Autodesk Fusion 360 part; units mm, degrees
sketch "Sketch1" plane through (0, 0, 0) normal (0, 0, 1) x (1, 0, 0)
  line L0 (12.2, 9.5) -> (-12.2, 9.5)
  line L1 (-12.2, 9.5) -> (-12.2, -9.5)
  line L2 (-12.2, -9.5) -> (12.2, -9.5)
  line L3 (12.2, -9.5) -> (12.2, 9.5)
  line L4 (12.2, 9.5) -> (-12.2, -9.5) construction
  line L5 (-12.2, 9.5) -> (12.2, -9.5) construction
  line L6 (9.2, 6.5) -> (-9.2, 6.5) construction
  line L7 (-9.2, 6.5) -> (-9.2, -6.5) construction
  line L8 (-9.2, -6.5) -> (9.2, -6.5) construction
  line L9 (9.2, -6.5) -> (9.2, 6.5) construction
  line L10 (9.2, 6.5) -> (-9.2, -6.5) construction
  line L11 (-9.2, 6.5) -> (9.2, -6.5) construction
  circle A0 centre (9.2, 6.5) radius 1.5
  circle A1 centre (-9.2, -6.5) radius 1.5
  line L12 (0, 0) -> (9.2, 0) construction
  circle A2 centre (-9.2, 6.5) radius 1.5
  circle A3 centre (9.2, -6.5) radius 1.5
  line L13 (6.2, 7.5) -> (-6.2, 7.5)
  line L14 (-6.2, 7.5) -> (-6.2, -7.5)
  line L15 (-6.2, -7.5) -> (6.2, -7.5)
  line L16 (6.2, -7.5) -> (6.2, 7.5)
  line L17 (6.2, 7.5) -> (-6.2, -7.5) construction
  line L18 (-6.2, 7.5) -> (6.2, -7.5) construction
  line L19 (0, 0) -> (5.0501, 0) construction
  line L20 (19.3001, 18.69) -> (-9.2, 18.69) construction
  line L21 (-9.2, 18.69) -> (-9.2, -18.69) construction
  line L22 (-9.2, -18.69) -> (19.3001, -18.69) construction
  line L23 (19.3001, -18.69) -> (19.3001, 18.69) construction
  line L24 (19.3001, 18.69) -> (-9.2, -18.69) construction
  line L25 (-9.2, 18.69) -> (19.3001, -18.69) construction
  circle A4 centre (-9.2, 18.69) radius 1.5
  circle A5 centre (-9.2, -18.69) radius 1.5
  line L26 (-12.2, 21.69) -> (-4.2, 21.69)
  line L27 (-4.2, 21.69) -> (-4.2, -21.69)
  line L28 (-4.2, -21.69) -> (-12.2, -21.69)
  line L29 (-12.2, -21.69) -> (-12.2, 21.69)
  point P0 (5.0501, 0)
  dimension "d1" = 18.4
  dimension "d2" = 13
  dimension "d3" = 3
  dimension "d6" = 3
  dimension "d7" = 3
  dimension "d10" = 3
  dimension "d11" = 2
  dimension "d14" = 37.38
  dimension "d15" = 3
  dimension "d16" = 3
  dimension "d17" = 5
  dimension "d18" = 3
  dimension "d19" = 3
extrude "Extrude1" add sketch "Sketch1" along normal blind 12 contours L0 L2 L3 L13 L15 L16 L27 | L0 L1 L2 L13 L14 L15 L27 L29
fillet "Fillet1" radius 2 4 edges at (12.2, -9.5, 6) (12.2, 9.5, 6) (-12.2, 9.5, 6) (-12.2, -9.5, 6)
thread "Thread1"
sketch "Sketch2" plane through (0, 0, 12) normal (0, 0, 1) x (1, 0, 0)
  line L0 (-12.2, 7.5) -> (-12.2, -7.5)
  line L1 (-10.2, -9.5) -> (10.2, -9.5)
  arc A0 (10.2, -9.5) -> (12.2, -7.5) centre (10.2, -7.5) ccw
  line L2 (12.2, -7.5) -> (12.2, 7.5)
  arc A1 (12.2, 7.5) -> (10.2, 9.5) centre (10.2, 7.5) ccw
  line L3 (10.2, 9.5) -> (-10.2, 9.5)
  line L4 (6.2, 7.5) -> (6.2, -7.5)
  line L5 (6.2, -7.5) -> (-6.2, -7.5)
  line L6 (-6.2, -7.5) -> (-6.2, 7.5)
  line L7 (-6.2, 7.5) -> (6.2, 7.5)
  circle A2 centre (9.2, 6.5) radius 1.2645
  circle A3 centre (-9.2, -6.5) radius 1.2645
  circle A4 centre (9.2, -6.5) radius 1.2645
  circle A5 centre (-9.2, 6.5) radius 1.2645
  line L8 (-12.2, -9.5) -> (-4.2, -9.5)
  line L9 (-4.2, -9.5) -> (-4.2, -14.69)
  line L10 (-4.2, -14.69) -> (-12.2, -14.69)
  line L11 (-12.2, -14.69) -> (-12.2, -9.5)
  line L12 (-4.2, -9.5) -> (-10.2, -9.5)
  line L13 (-4.2, -14.69) -> (-12.2, -14.69)
  line L14 (-12.2, -14.69) -> (-12.2, -11.69)
  line L15 (-12.2, -11.69) -> (-4.2, -11.69)
  line L16 (-4.2, -11.69) -> (-4.2, -14.69)
  line L17 (0, 0) -> (12.2, 0)
  line L18 (-12.2, 14.69) -> (-12.2, 9.5)
  line L19 (-12.2, 9.5) -> (-4.2, 9.5)
  line L20 (-4.2, 14.69) -> (-12.2, 14.69)
  line L21 (-12.2, 14.69) -> (-12.2, 11.69)
  line L22 (-4.2, 11.69) -> (-4.2, 14.69)
  line L23 (-12.2, 11.69) -> (-4.2, 11.69)
  line L24 (-4.2, 9.5) -> (-4.2, 14.69)
  line L25 (-4.2, 9.5) -> (-10.2, 9.5)
  arc A6 (-12.2, -7.5) -> (-10.2, -9.5) centre (-10.2, -7.5) ccw
  arc A7 (-10.2, 9.5) -> (-12.2, 7.5) centre (-10.2, 7.5) ccw
  dimension "d23" = 3
chamfer "Chamfer1" distance 0.5 angle 45 8 edges at (12.2, 0, 12) (11.6142, 8.9142, 12) (0, 9.5, 12) (-11.6142, 8.9142, 12) (-12.2, 0, 12) (-11.6142, -8.9142, 12) (0, -9.5, 12) (11.6142, -8.9142, 12)
equation "d19 = d18"
Can you work these out from the model? Positions are in its coordinate system, mm. A direction names the side the tool comes from. Round coordinates to 2 decimals unless told otherwise and drop trailing zeros. Write each loop counter-clockwise with the first axis right and the second up, starting at its lowest first coordinate (ties: lowest second). Pieces come first, ordered by that corner, then holes. Notation, with made-up numbers: (41.5, 88.25) -> (65.5, 88.25) arc R23 ccw to (65.5, 125.25) -> close; hole circle Ø4 at (13.25, -30). An arc over 180 degrees is marked (long way). Use one line per item in the form item = value. Start each with the question number.
Q1. Imagine slicing it at D-D (x = -3). Please give me the cut outline in (y, z).
Q2. We'd pull the mould along X, two halves only. Please class faces 1 (the face through (-8, 0, 0)), 2 (the face through (-7.814, 7.075, 5.916)), 3 (the face through (11.6, -8.93, 5.83)), 4 (the face through (-11.6, 8.93, 5.83)): +X half, -X half, draft (parallel to the pull), parting line (faces both ways), or undercut.
Q3. Imagine slicing it at B-B (x = 9.2). Please give me the cut outline in (y, z), then the cut area to 3 significant figures.
Q4. I'm going to push a flat-ended pin straight in: P1, Ø4, axis at x = -9.2, y = 6.5, coming from the +Z side. Where does the tip first touch, or does it pass through?
Q5. Which directions (+Z, -Z, +X, -X, +Y, -Y) give clear straight access to the entire face, cutting with the end or side of a thin tool? Please do faces 5 (the face through (0, -9.5, 6)), 6 (the face through (-6.2, 0, 6)).
Q6. Imagine slicing it at A-A (y = -2.5). Please give me the cut outline in (x, z).
Q7. If I drill on probe 1 along Y at (x, z) = (9.2, 3); probe 2 along X at (y, z) = (4.75, 7.5); probe 3 along X at (y, z) = (-7, 3.25), over which ranges is the centre line in solid material (lowest first)? Write a range as [from, to].
Q8. Imagine slicing it at C-C (y = -6.5). Please give me the cut outline in (x, z), then the cut area to 4 significant figures.
Worked out:
q1.outline = (-9.5, 0) -> (-7.5, 0) -> (-7.5, 12) -> (-9, 12) -> (-9.5, 11.5) -> close; (7.5, 0) -> (9.5, 0) -> (9.5, 11.5) -> (9, 12) -> (7.5, 12) -> close
q2.face_1 = draft
q2.face_2 = undercut
q2.face_3 = +X half
q2.face_4 = -X half
q3.outline = (-9.5, 0) -> (-8, 0) -> (-8, 12) -> (-9, 12) -> (-9.5, 11.5) -> close; (-5, 0) -> (5, 0) -> (5, 12) -> (-5, 12) -> close; (8, 0) -> (9.5, 0) -> (9.5, 11.5) -> (9, 12) -> (8, 12) -> close
q3.area = 156 mm^2
q4.P1 = 12
q5.face_5 = +Z, -Z, +X, -X, -Y
q5.face_6 = +Z, -Z
q6.outline = (-12.2, 0) -> (-6.2, 0) -> (-6.2, 12) -> (-11.7, 12) -> (-12.2, 11.5) -> close; (6.2, 0) -> (12.2, 0) -> (12.2, 11.5) -> (11.7, 12) -> (6.2, 12) -> close
q7.probe_1 = [-9.5, -8], [-5, 5], [8, 9.5]
q7.probe_2 = [-12.2, -6.2], [6.2, 12.2]
q7.probe_3 = [-12.2, -10.61], [-7.79, -6.2], [6.2, 7.79], [10.61, 12.2]
q8.outline = (-12.2, 0) -> (-10.7, 0) -> (-10.7, 12) -> (-11.7, 12) -> (-12.2, 11.5) -> close; (-7.7, 0) -> (-6.2, 0) -> (-6.2, 12) -> (-7.7, 12) -> close; (6.2, 0) -> (7.7, 0) -> (7.7, 12) -> (6.2, 12) -> close; (10.7, 0) -> (12.2, 0) -> (12.2, 11.5) -> (11.7, 12) -> (10.7, 12) -> close
q8.area = 71.75 mm^2
